Answer from the drawing. Dimensions are ordinates in mm from the lowest x, y and z of the part. Give positions to 0.01 mm unless a question says otherwise; leave off trailing zeros. Order: outer loops, then holes, each group sorted by start corner. A loop starts at its lowest first (then second) coordinate and runs counter-clockwise, first axis right, second up.
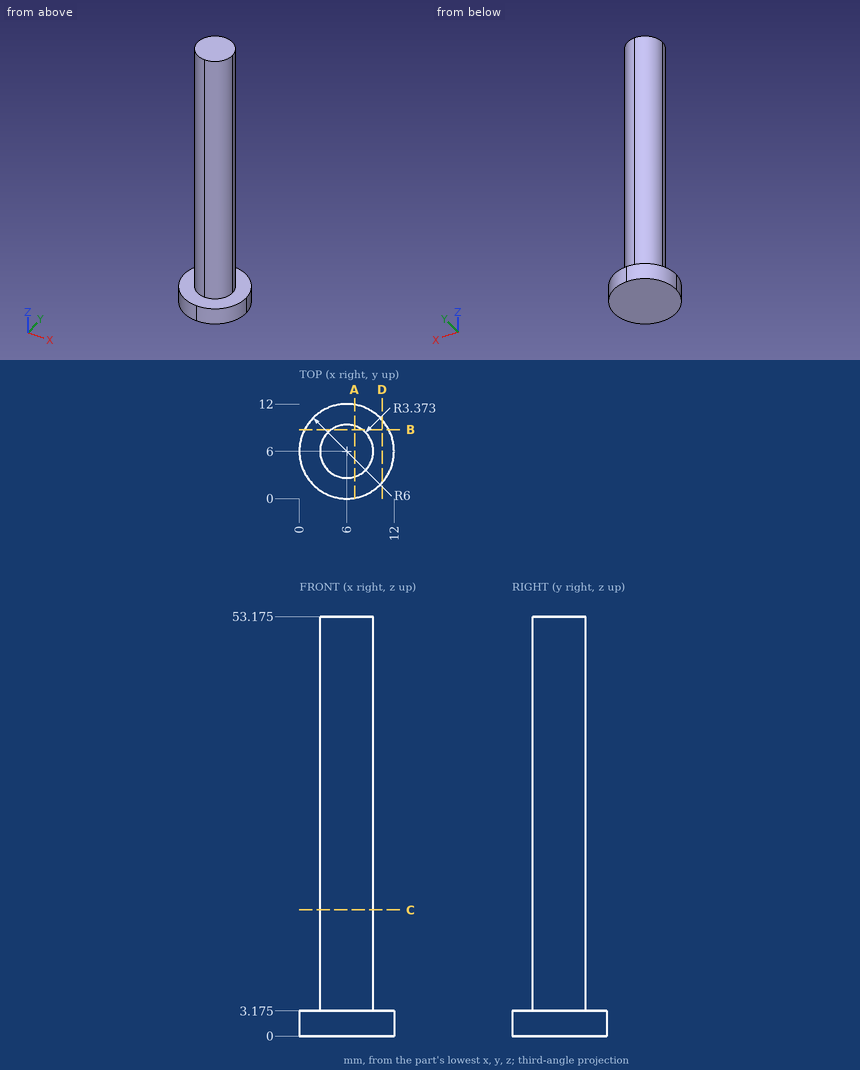
1. The part is cut by section A-A (x = 7). Write down the section's boundary in (y, z) (1 decimal), then the cut area to 3 significant figures.
Findings below:
outline: (0.1, 0) - (11.9, 0) - (11.9, 3.2) - (9.2, 3.2) - (9.2, 53.2) - (2.8, 53.2) - (2.8, 3.2) - (0.1, 3.2) - close
area: 360 mm2
2. The part is cut by section D-D (x = 10.5). Write down the section's boundary in (y, z) (1 decimal).
Findings below:
outline: (2, 0) - (10, 0) - (10, 3.2) - (2, 3.2) - close
3. Given P1, Ø4, axis at x = 7.5, z = 37, coming from the +Y side; P2, Ø5, axis at y = 3.5, z = 13.5, coming from the +X side; P3, Ø4, axis at y = 6.5, z = 32, coming from the -X side, each flat-ended and moving along its own axis, determine where each tip first touches the part or whether it passes through.
Findings below:
P1: stops at y = 9.37
P2: stops at x = 9.37
P3: stops at x = 2.63
4. Straight lines are drawn through the part: probe 1 along Y at (x, z) = (5.75, 34) (1 decimal); probe 2 along Z at (x, y) = (3.25, 1.25) (1 decimal); probe 3 along X at (y, z) = (8.5, 16.5) (1 decimal). For each, find the intervals that lie inside material, in ascending order.
Findings below:
probe 1: y = 2.6 to 9.4
probe 2: z = 0 to 3.2
probe 3: x = 3.7 to 8.3
5. The part is cut by section C-C (z = 16). Write down the section's boundary in (x, y).
Findings below:
outline: circle Ø6.75 at (6, 6)
6. The part is cut by section B-B (y = 8.75). Write down the section's boundary in (x, z) (1 decimal), then the cut area to 3 significant figures.
Findings below:
outline: (0.7, 0) - (11.3, 0) - (11.3, 3.2) - (8, 3.2) - (8, 53.2) - (4, 53.2) - (4, 3.2) - (0.7, 3.2) - close
area: 229 mm2
